Can you work these out from the model? Positions are in its coordinate system, mm. A direction names the side the tool comes from. Give positions to 0.01 mm unless a question says otherwise; leave off trailing zeros. Order: outer loops, then holes, each group sorted by start corner. A loop starts at its lowest first (then second) coordinate and runs counter-clockwise, first axis right, second up. Notation, with made-up numbers: M 49,6 L 95,6 A10 ccw 95,16 Z; hole C 77.5,83 d4. An arc over 180 degrees is marked long. One line per question, with ' | ' between items. Start each with the question number.
1) If we section it at A-A, the plane y = 12: Please give me the cut outline in (x, z), plus the area to 3 significant figures.
2) Thinking about a two-plate mould opening in X: for faces 1 (the flat face through (0, 59.1, 0)), 2 (the flat face through (11.25, -3, 0)), 3 (the cylindrical face through (4.96, 41.67, 4.61)), which applies, +X half, -X half, draft (parallel to the pull), parting line (faces both ways), or undercut?
3) Please list where these lines run through material, in increasing order: line 1 along X through (y, z) = (45.3, 0); line 2 along Y through (x, z) = (-9.75, -1.5); line 3 along Z through (x, y) = (-8.5, 39.5). Write a range as [from, to].
4) If we section it at B-B, the plane y = 27: Please give me the cut outline in (x, z).
5) I'm going to push flat-ended pins straight in: pin 1 Ø3 at (x, y) = (3.5, 45) entering from +Z; pin 2 Ø1.5 at (x, z) = (8, 2.5) entering from +Y; pin 3 Ø0.6 at (x, y) = (11, -2.5) entering from +Z. Where does each tip first touch, or does it pass through?
6) For faces 4 (the cylindrical face through (8.9, 41.53, 3.48)), 5 (the cylindrical face through (-2.579, -3.193, 1.978)), which set-ups out of +Z, -Z, +X, -X, +Y, -Y let a thin tool reach every point of the face, with its end or its side?
7) If we section it at C-C, the plane y = 53.5: Please give me the cut outline in (x, z), plus the area to 3 significant figures.
Autodesk Inventor part; units mm, degrees
ref_plane "Work Plane1" through (0, 41.6, 0) normal (0, 1, 0) x (1, 0, 0)
ref_plane "Work Plane2" through (0, 50.6, 0) normal (0, 1, 0) x (1, 0, 0)
ref_plane "YZ Plane" through (0, 0, 0) normal (1, 0, 0) x (0, 1, 0)
sketch "Sketch1" plane through (0, 0, 0) normal (0, 1, 0) x (-1, 0, 0)
  circle A0 centre (0, 0) radius 14
  dimension "d0" = 28
extrude "Extrusion1" add sketch "Sketch1" along normal blind 46.6
sketch "Sketch2" plane through (0, 46.6, 0) normal (0, 1, 0) x (1, 0, 0)
  circle A0 centre (0, 0) radius 14
  circle A1 centre (0, 0) radius 5
  dimension "d3" = 10
extrude "Extrusion2" add sketch "Sketch2" along normal blind 3 contours A1
sketch "Sketch3" plane through (0, 46.6, 0) normal (0, 1, 0) x (1, 0, 0)
  circle A0 centre (0, 0) radius 5
  circle A1 centre (0, 0) radius 5
  circle A2 centre (0, 0) radius 14
  circle A3 centre (0, 0) radius 14
  line L0 (-14, 0) -> (14, 0)
  point P0 (-8, 0)
  point P1 (8, 0)
  dimension "d6" = 16
  dimension "d7" = 6
  dimension "d8" = 6
hole "Hole1" at (-8, 46.6, 0) at (8, 46.6, 0) direction (0, -1, 0) diameter 2.459 depth 3
ref_plane "Work Plane1" through (0, 41.6, 0) normal (0, 1, 0) x (1, 0, 0)
sketch "Sketch4" plane through (0, 41.6, 0) normal (0, 1, 0) x (1, 0, 0)
  circle A0 centre (0, 0) radius 15
  dimension "d17" = 30
extrude "Extrusion3" add sketch "Sketch4" against normal blind 27.7
sketch "Sketch5" plane through (0, 0, 0) normal (0, -1, 0) x (1, 0, 0)
  circle A0 centre (0, 0) radius 5
  dimension "d20" = 10
extrude "Extrusion4" add sketch "Sketch5" along normal blind 2.7
sketch "Sketch6" plane through (0, 0, 0) normal (0, -1, 0) x (1, 0, 0)
  circle A0 centre (0, 0) radius 5
  circle A1 centre (0, 0) radius 5
  circle A2 centre (0, 0) radius 14
  circle A3 centre (0, 0) radius 14
  line L0 (14, 0) -> (-14, 0)
  line L1 (-11.25, 1.35) -> (-11.75, 1.35)
  line L2 (-11.75, 1.35) -> (-11.75, -1.35)
  line L3 (-11.75, -1.35) -> (-11.25, -1.35)
  line L4 (-11.25, -1.35) -> (-11.25, 1.35)
  line L5 (11.25, 1.35) -> (10.75, 1.35)
  line L6 (10.75, 1.35) -> (10.75, -1.35)
  line L7 (10.75, -1.35) -> (11.25, -1.35)
  line L8 (11.25, -1.35) -> (11.25, 1.35)
  dimension "d23" = 22
  dimension "d24" = 0.5
  dimension "d25" = 0.5
  dimension "d26" = 11.25
  dimension "d27" = 11.25
  dimension "d28" = 2.7
  dimension "d29" = 2.7
  dimension "d30" = 1.35
  dimension "d31" = 1.35
extrude "Extrusion5" add sketch "Sketch6" along normal blind 5.5 contours L6 L5 L8 L0 | L0 L8 L7 L6 | L4 L3 L2 L0 | L0 L2 L1 L4
sketch "Sketch7" plane through (0, 49.6, 0) normal (0, 1, 0) x (1, 0, 0)
  circle A0 centre (0, 0) radius 1.15
  dimension "d34" = 2.3
extrude "Extrusion6" add sketch "Sketch7" along normal blind 9.5
ref_plane "Work Plane2" through (0, 50.6, 0) normal (0, 1, 0) x (1, 0, 0)
sketch "Sketch10" plane through (0, 0, 0) normal (1, 0, 0) x (0, 1, 0)
  line L0 (0, -14) -> (0, 14)
  line L1 (13.9, 14) -> (13.9, -14)
  line L2 (8.5, 3.8) -> (13.9, 3.8)
  line L3 (13.9, 3.8) -> (13.9, -3.8)
  line L4 (13.9, -3.8) -> (8.5, -3.8)
  line L5 (8.5, -3.8) -> (8.5, 3.8)
  circle A0 centre (11.2, 3.8) radius 2.7
  circle A1 centre (11.2, -3.8) radius 2.7
  line L6 (0, 0) -> (13.9, 0)
  line L7 (13.9, 14) -> (13.9, -14)
  line L8 (0, -14) -> (13.9, -14)
  point P0 (11.2, -6.5)
  point P1 (11.2, 6.5)
  dimension "d57" = 8.5
  dimension "d59" = 0
  dimension "d60" = 5.4
  dimension "d61" = 13.9
  dimension "d65" = 3.8
  dimension "d66" = 3.8
  dimension "d80" = 5.4
  dimension "d81" = 5.4
  dimension "d82" = 2.7
  dimension "d83" = 2.7
  dimension "d84" = 13
extrude "Extrusion9" cut sketch "Sketch10" along normal mid plane 31.5 contours L6 L1 A1 L5 | L5 A0 L1 L6 | A1 L4 | L4 A1 | A0 L2 | L2 A0
sketch "Sketch12" plane through (0, 46.6, 0) normal (0, 1, 0) x (1, 0, 0)
  circle A0 centre (0, 0) radius 1.15
  circle A1 centre (0, 0) radius 5
  circle A2 centre (-8, 0) radius 1.2295
  circle A3 centre (8, 0) radius 1.2295
  circle A4 centre (0, 0) radius 5
  circle A5 centre (0, 0) radius 14
  circle A6 centre (0, 0) radius 14
  line L0 (-14, 0) -> (14, 0)
  line L1 (0, 14) -> (0, -14)
  circle A7 centre (0, 0) radius 6.7705
  circle A8 centre (0, 0) radius 9.8705
  line L2 (-2.75, 6.1869) -> (-4.0091, 9.0196)
  line L3 (-6.3854, 2.2508) -> (-9.3091, 3.2814)
  line L4 (2.75, 6.1869) -> (4.0091, 9.0196)
  line L5 (6.3854, 2.2508) -> (9.3091, 3.2814)
  circle A9 centre (-8, 0) radius 1.2295
  circle A10 centre (8, 0) radius 1.2295
  line L6 (-2.75, -6.1869) -> (-4.0091, -9.0196)
  line L7 (-6.3854, -2.2508) -> (-9.3091, -3.2814)
  line L8 (2.75, -6.1869) -> (4.0091, -9.0196)
  line L9 (6.3854, -2.2508) -> (9.3091, -3.2814)
  point P0 (0, 6.7705)
  point P1 (0, 9.8705)
  point P2 (-8, 1.2295)
  point P3 (8, 1.2295)
  point P4 (-6.3854, -2.2508)
  point P5 (6.3854, -2.2508)
  dimension "d85" = 3.1
  dimension "d86" = 5.5
  dimension "d87" = 4.0091
  dimension "d88" = 4.0091
  dimension "d89" = 1.5
  dimension "d90" = 1.5
  dimension "d91" = 1.2295
  dimension "d92" = 2.459
  dimension "d93" = 2.459
  dimension "d94" = 1.2295
extrude "Extrusion11" cut sketch "Sketch12" against normal blind 10 contours A7 L4 A8 L5 | L9 A8 L8 A7 | A7 L3 A8 L2 | L6 A8 L7 A7
fillet "Fillet1" radius 1 16 edges at (-4.0091, 41.6, -9.0196) (-2.75, 41.6, -6.1869) (-6.3854, 41.6, -2.2508) (-9.3091, 41.6, -3.2814) (9.3091, 41.6, -3.2814) (6.3854, 41.6, -2.2508) (4.0091, 41.6, -9.0196) (9.3091, 41.6, 3.2814) (6.3854, 41.6, 2.2508) (4.0091, 41.6, 9.0196) (2.75, 41.6, 6.1869) (-4.0091, 41.6, 9.0196) (-9.3091, 41.6, 3.2814) (-6.3854, 41.6, 2.2508) (-2.75, 41.6, 6.1869) (2.75, 41.6, -6.1869)
sketch "Sketch13" plane through (0, -2.7, 0) normal (0, -1, 0) x (1, 0, 0)
  circle A0 centre (0, 0) radius 3.25
  dimension "d98" = 6.5
extrude "Extrusion12" add sketch "Sketch13" along normal blind 1
sketch "Sketch14" plane through (0, -3.7, 0) normal (0, -1, 0) x (1, 0, 0)
  circle A0 centre (0, 0) radius 1.2
  dimension "d101" = 2.4
extrude "Extrusion13" add sketch "Sketch14" along normal blind 1.1
equation "\"d26\" = d27"
equation "\"d30\" = d31"
equation "\"d65\" = d66"
equation "\"d82\" = 0.5 * d80"
equation "\"d83\" = 0.5 * d81"
equation "\"d87\" = d88"
equation "\"d41\" = d42"
properties part number "rs390" material "Steel, Mild"
Results found:
1) outline: M -12.46,-6.38 A14 ccw 12.46,-6.38 Z; M -12.46,6.38 L 12.46,6.38 A14 ccw Z | area: 271 mm²
2) face 1: draft | face 2: +X half | face 3: undercut
3) line 1: x = [-14, -9.23], [-6.77, 6.77], [9.23, 14] | line 2: y = [0, 8.5], [13.9, 46.6] | line 3: z = [-12.36, -5.02], [-3.02, 3.02], [5.02, 12.36]
4) outline: C 0,0 d30
5) pin 1: stops at z = 13.86 | pin 2: stops at y = 46.6 | pin 3: stops at z = 1.35
6) face 4: +Y | face 5: -Y
7) outline: C 0,0 d2.3 | area: 4.15 mm²
